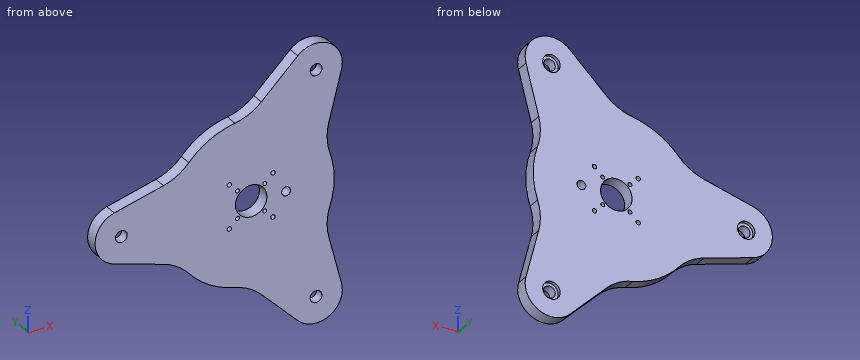
from build123d import *

# Parameters (mm, degrees)
SKETCH1_R                = 95
BOSS_EXTRUDE1_DEPTH      = 15
SKETCH2_R                = 10
BOSS_EXTRUDE2_DEPTH      = 15
FILLET1_R                = 60
SKETCH4_R                = 10
BOSS_EXTRUDE3_DEPTH      = 11
M12_CLEARANCE_HOLE1_D    = 13.5
CIRPATTERN1_COUNT        = 3
FILLET1_OF_CIRPATTERN1_R = 60
SKETCH7_R                = 18
CUT_EXTRUDE1_DEPTH       = 240.25451688
M4_CLEARANCE_HOLE1_D     = 4.5
M6_TAPPED_HOLE1_D        = 5
M12_TAPPED_HOLE1_D       = 10.2


with BuildPart() as part:
    # Sketch1 → Boss-Extrude1 (new body)
    with BuildSketch(Plane(origin=(0, 0, 0), x_dir=(1, 0, 0), z_dir=(0, 1, 0))):
        with Locations(Location((0, 0, 0), (0, 0, 270))):
            Circle(SKETCH1_R)
    extrude(amount=BOSS_EXTRUDE1_DEPTH)

    # Sketch2 → Boss-Extrude2 (add)
    with BuildSketch(Plane.XZ):
        with BuildLine():
            Line((-156.547830163, -28.900388054), (-80.777472107, -50))
            ThreePointArc((-80.777472107, -50), (-95, 0), (-80.777472107, 50))
            Line((-80.777472107, 50), (-156.547830163, 28.900388054))
            ThreePointArc((-156.547830163, 28.900388054), (-178.5, 0), (-156.547830163, -28.900388054))
        make_face()
        with Locations(Location((-148.5, 0, 0), (0, 0, 270))):
            Circle(SKETCH2_R, mode=Mode.SUBTRACT)
    boss_extrude2 = extrude(amount=-BOSS_EXTRUDE2_DEPTH)

    # Fillet1
    fillet1_edges = [part.edges().sort_by_distance(p)[0] for p in [
        (-80.777472107, 7.5, 50),
        (-80.777472107, 7.5, -50),
    ]]
    fillet(fillet1_edges, radius=FILLET1_R)

    # Sketch4 → Boss-Extrude3 (add)
    with BuildSketch(Plane.XZ):
        with Locations(Location((-148.5, 0, 0), (0, 0, 271.879376726))):
            Circle(SKETCH4_R)
    boss_extrude3 = extrude(amount=-BOSS_EXTRUDE3_DEPTH)

    # M12 Clearance Hole1 (through all)
    with Locations(Plane(origin=(0, 0, 0), x_dir=(-1, 0, 0), z_dir=(0, -1, 0))):
        with Locations((148.5, 0)):
            m12_clearance_hole1 = Hole(M12_CLEARANCE_HOLE1_D / 2)

    # CirPattern1: Boss-Extrude2, Boss-Extrude3, M12 Clearance Hole1 ×3 about axis
    cirpattern1_axis = Axis((0, 0, 0), (0, 1, 0))
    add([boss_extrude2.rotate(cirpattern1_axis, i * 360 / CIRPATTERN1_COUNT) for i in range(1, CIRPATTERN1_COUNT)])
    add([boss_extrude3.rotate(cirpattern1_axis, i * 360 / CIRPATTERN1_COUNT) for i in range(1, CIRPATTERN1_COUNT)])
    add([m12_clearance_hole1.rotate(cirpattern1_axis, i * 360 / CIRPATTERN1_COUNT) for i in range(1, CIRPATTERN1_COUNT)], mode=Mode.SUBTRACT)

    # Fillet1 of CirPattern1
    fillet1_of_cirpattern1_edges = [part.edges().sort_by_distance(p)[0] for p in [
        (83.690006243, 7.5, 44.955342898),
        (-2.912534136, 7.5, 94.955342898),
        (-2.912534136, 7.5, -94.955342898),
        (83.690006243, 7.5, -44.955342898),
    ]]
    fillet(fillet1_of_cirpattern1_edges, radius=FILLET1_OF_CIRPATTERN1_R)

    # Sketch7 → Cut-Extrude1 (cut, through all)
    with BuildSketch(Plane(origin=(0, 0, 0), x_dir=(-1, 0, 0), z_dir=(0, -1, 0))):
        with Locations(Location((0, 0, 0), (0, 0, 90))):
            Circle(SKETCH7_R)
    extrude(amount=-CUT_EXTRUDE1_DEPTH, mode=Mode.SUBTRACT)

    # M4 Clearance Hole1 (through all)
    with Locations(Plane(origin=(0, 15, 0), x_dir=(1, 0, 0), z_dir=(0, 1, 0))):
        with Locations((-15.556349186, -15.556349186), (15.556349186, -15.556349186), (15.556349186, 15.556349186), (-15.556349186, 15.556349186)):
            Hole(M4_CLEARANCE_HOLE1_D / 2)

    # M6 Tapped Hole1 (through all)
    with Locations(Plane(origin=(0, 0, 0), x_dir=(-1, 0, 0), z_dir=(0, -1, 0))):
        with Locations((0, 0), (25, 25), (-25, -25), (-25, 25), (25, -25)):
            Hole(M6_TAPPED_HOLE1_D / 2)

    # M12 Tapped Hole1 (through all)
    with Locations(Plane(origin=(0, 15, 0), x_dir=(1, 0, 0), z_dir=(0, 1, 0))):
        with Locations((40, 0)):
            Hole(M12_TAPPED_HOLE1_D / 2)


solid = part.part
Can you work these out from the model? Positions are in its coordinate system, mm. Coordinates: 2 decimals unless noted, no trailing zeros. Loops run counter-clockwise (first coordinate to the right, second up) from the corner with the lowest first, then second, coordinate; pieces in that order, holes last. Notation, with made-up numbers: M 54,43.25 L 84,43.25 A24 ccw 84,81.25 Z; hole C 8.5,-3 d8. An arc over 180 degrees is marked long. Answer as CSV lines item,"result". Start each with the question number.
1. Suppose I cut it at B-B, the plane x = -4.5. List the corners of the cut face in (y, z) for me.
2. Suppose I cut it at D-D, the plane x = -148.5. List the corners of the cut face in (y, z) for me, plus the area to 3 significant figures.
3. If I drill on probe 1 along Z at (x, y) = (74.25, 5.75); probe 2 along Z at (x, y) = (70.5, 3.25); probe 3 along X at (y, z) = (9, -25), over which ranges is the centre line in solid material (lowest first)? Write a range as [from, to].
4. Suppose I cut it at C-C, the plane y = 3.5. Count the separate pieces of the cut face and the enclosed holes in it, plus the area to 3 significant figures.
5. For pin 1 Ø2.5 at (x, z) = (15.56, 15.56) entering from -Y; pin 2 Ø3 at (y, z) = (8.5, 76) entering from -X; pin 3 Ø6 at (y, z) = (12, -102) entering from +X; pin 4 Ø4 at (y, z) = (4.5, -6) entering from -X, each with a flat end and sliding along its axis, tell me the tip position at first contact or that it passes through.
6. Suppose I cut it at A-A, the plane z = 0. List the corners of the cut face in (x, y) for me.
Output:
1,outline,"M 0,-97.88 L 15,-97.88 L 15,-17.43 L 0,-17.43 Z; M 0,17.43 L 15,17.43 L 15,97.88 L 0,97.88 Z"
2,outline,"M 0,-31.14 L 15,-31.14 L 15,-10 L 11,-10 L 11,-6.75 L 0,-6.75 Z; M 0,6.75 L 11,6.75 L 11,10 L 15,10 L 15,31.14 L 0,31.14 Z"
2,area,"706 mm^2"
3,probe 1,"z = [-158.6, -135.35], [-121.85, 121.85], [135.35, 158.6]"
3,probe 2,"z = [-158.37, -134.22], [-122.99, 122.99], [134.22, 158.37]"
3,probe 3,"x = [-165.08, -27.5], [-22.5, 22.5], [27.5, 91.65]"
4,separate pieces,"1"
4,enclosed holes,"13"
4,area,"44,800 mm^2"
5,pin 1,"passes through"
5,pin 2,"stops at x = -58.95"
5,pin 3,"stops at x = 99.15"
5,pin 4,"stops at x = -178.23"
6,outline,"M -178.5,0 L -155.25,0 L -155.25,11 L -158.5,11 L -158.5,15 L -178.5,15 Z; M -141.75,0 L -18,0 L -18,15 L -138.5,15 L -138.5,11 L -141.75,11 Z; M 18,0 L 34.9,0 L 34.9,15 L 18,15 Z; M 45.1,0 L 95,0 L 95,15 L 45.1,15 Z"
